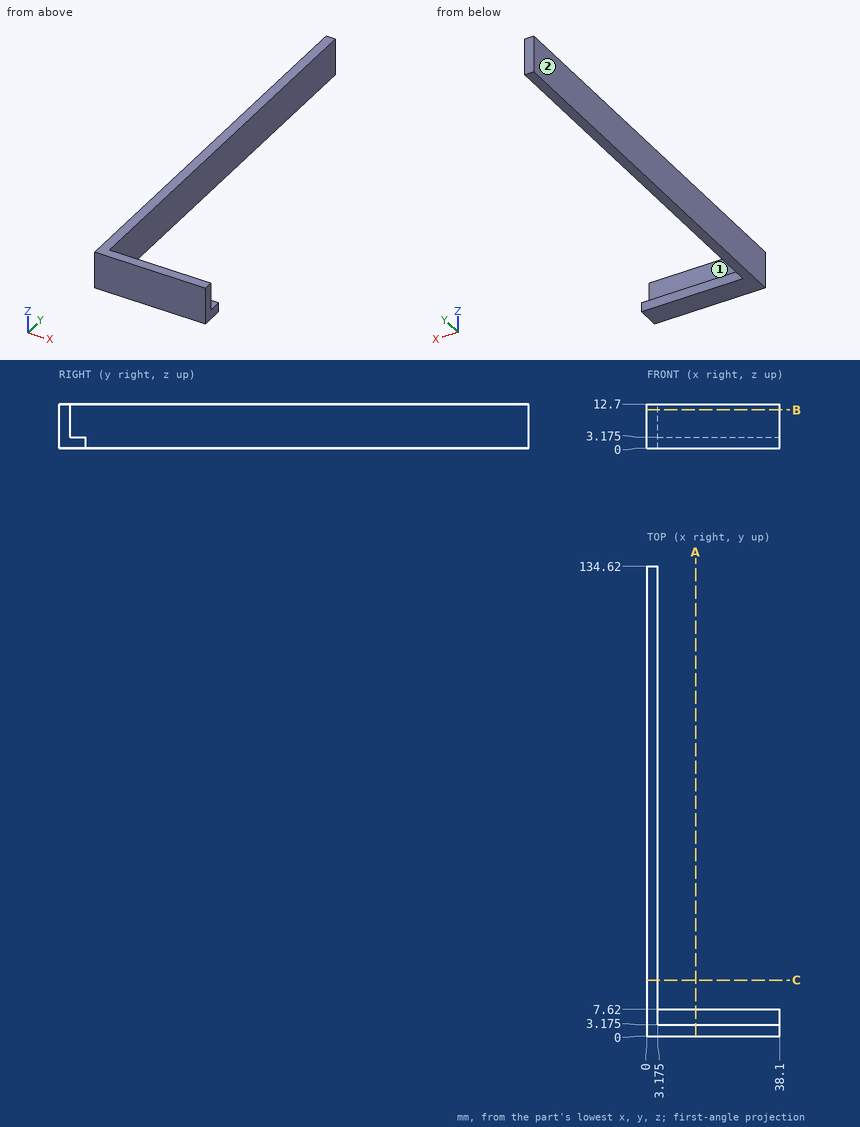
The figure shows three views and two pictorial views of one solid part (mm, origin at its lowest corner). Answer the questions. A direction names the side the tool comes from. Round coordinates to 2 decimals unless told otherwise and drop trailing zeros. Write each loop counter-clockwise with the first axis right and the second up, starting at its lowest first coordinate (ties: lowest second). Pieces come first, ordered by that corner, then holes. Notation, with made-up numbers: (2.5, 34) - (28.5, 34) arc R14 cw to (28.5, 50) - close; hole circle Ø6 at (78.25, 45). An arc over 180 degrees is marked (long way). Answer in a Markdown table with one row per item. Add a question column.
1. A cutting plane is placed at B-B, the plane z = 11. Determine the outline of the cut face in (x, y) (3 decimals).
2. A cutting plane is placed at A-A, the plane x = 14. Determine the outline of the cut face in (y, z) (3 decimals), and give its area (3 significant figures).
3. Given pin 1 (2.5 mm diameter, centred on x = 12, z = 1.5, fed in from +Y); pin 2 (1.5 mm diameter, centred on y = 27.5, z = 11, fed in from +X) (3 decimals); pin 3 (5 mm diameter, centred on x = 19, y = 6, fed in from +Z) (3 decimals), each flat-ended and moving along its own axis, determine where each tip first touches the part or whether it passes through.
4. For the marked faces 1 and 2, determine the directions among +Z, -Z, +X, -X, +Y, -Y from which every point of the face is accessible in a straight line to the end or side of a thin tool.
5. Find the intervals of material crossed by line 1 along Y through (x, z) = (7.5, 5.25) (3 decimals); line 2 along Y through (x, z) = (7.5, 1.5), in increasing order. Write a range as from..to.
6. A cutting plane is placed at C-C, the plane y = 16. Determine the outline of the cut face in (x, z) (3 decimals).
Worked out:
| question | item | result |
|---|---|---|
| 1 | outline | (0, 0) - (38.1, 0) - (38.1, 3.175) - (3.175, 3.175) - (3.175, 134.62) - (0, 134.62) - close |
| 2 | outline | (0, 0) - (7.62, 0) - (7.62, 3.175) - (3.175, 3.175) - (3.175, 12.7) - (0, 12.7) - close |
| 2 | area | 54.4 mm^2 |
| 3 | pin 1 | y = 7.62 |
| 3 | pin 2 | x = 3.175 |
| 3 | pin 3 | z = 3.175 |
| 4 | face 1 | +Z, +X, +Y |
| 4 | face 2 | +Z, -Z, -X, +Y, -Y |
| 5 | line 1 | 0..3.175 |
| 5 | line 2 | 0..7.62 |
| 6 | outline | (0, 0) - (3.175, 0) - (3.175, 12.7) - (0, 12.7) - close |
